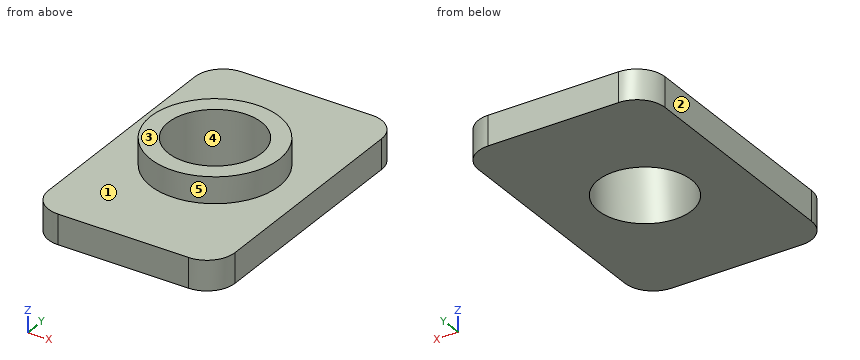
Autodesk Inventor part; units mm, degrees
ref_plane "YZ Plane" through (0, 0, 0) normal (1, 0, 0) x (0, 1, 0)
ref_plane "XZ Plane" through (0, 0, 0) normal (0, 1, 0) x (-1, 0, 0)
ref_plane "XY Plane" through (0, 0, 0) normal (0, 0, 1) x (1, 0, 0)
sketch "Sketch1" plane through (0, 0, 0) normal (0, 0, 1) x (1, 0, 0)
  line L0 (-5, 7.5) -> (5, 7.5)
  line L1 (5, 7.5) -> (5, -7.5)
  line L2 (5, -7.5) -> (-5, -7.5)
  line L3 (-5, -7.5) -> (-5, 7.5)
  line L4 (0, 7.5) -> (0, -7.5) construction
  line L5 (-5, 0) -> (5, 0) construction
  circle A0 centre (0, 0) radius 2.5
  dimension "d0" = 15
  dimension "d1" = 10
  dimension "d2" = 5
extrude "Extrusion1" add sketch "Sketch1" along normal blind 1.6
sketch "Sketch2" plane through (0, 0, 1.6) normal (0, 0, 1) x (1, 0, 0)
  circle A0 centre (0, 0) radius 2.5
  circle A1 centre (0, 0) radius 3.45
  dimension "d5" = 6.9
extrude "Extrusion2" add sketch "Sketch2" along normal blind 1.4
thread "Thread1"
fillet "Fillet1" radius 1.5 4 edges at (5, 7.5, 0.8) (-5, 7.5, 0.8) (-5, -7.5, 0.8) (5, -7.5, 0.8)
properties part number "t-nut"
Geometry check sheet. Reference: the model listing, model coordinates, mm. Face numbers are marked on the shaded views. A direction names the side the tool comes from. Coordinates: 2 decimals unless noted, no trailing zeros. Order: outer loops, then holes, each group sorted by start corner. A loop starts at its lowest first (then second) coordinate and runs counter-clockwise, first axis right, second up. Notation, with made-up numbers: M 65.25,60.5 L 72.25,60.5 A31 ccw 72.25,89.5 Z; hole C 45,63 d6. An arc over 180 degrees is marked long. Answer as a JSON object with one key per item and string values.
Q1. Tool access check on the marked faces 1 and 2. Record the directions out of +Z, -Z, +X, -X, +Y, -Y that give a thin tool (end or side, any length) a straight path to the whole face; none if there is none.
Results are:
{"face 1": "+Z", "face 2": "+Z, -Z, -X, +Y, -Y"}
Q2. Cross-section at C-C on z = 0.5. Record the cut outline in (x, y).
Results are:
{"outline": "M -5,-6 A1.5 ccw -3.5,-7.5 L 3.5,-7.5 A1.5 ccw 5,-6 L 5,6 A1.5 ccw 3.5,7.5 L -3.5,7.5 A1.5 ccw -5,6 Z; hole C 0,0 d5"}
Q3. Release check for a two-part mould opening along Y. For the marked faces 3, 4 and 5 record: released by +Y, released by -Y, zero draft, split by the parting line, or undercut.
Results are:
{"face 3": "zero draft", "face 4": "undercut", "face 5": "split by the parting line"}
Q4. Cross-section at D-D on y = -3. Record the cut outline in (x, z).
Results are:
{"outline": "M -5,0 L 5,0 L 5,1.6 L 1.7,1.6 L 1.7,3 L -1.7,3 L -1.7,1.6 L -5,1.6 Z"}
Q5. Scan lines: line 1 (Y direction, x = 0, z = 1.25); line 2 (Z direction, x = 0.5, y = -3.5); line 3 (Y direction, x = -2, z = 1.2). Record each from-to range of solid material in increasing order.
Results are:
{"line 1": "y = -7.5 to -2.5, 2.5 to 7.5", "line 2": "z = 0 to 1.6", "line 3": "y = -7.5 to -1.5, 1.5 to 7.5"}
Q6. Cross-section at A-A on y = 0. Record the cut outline in (x, z).
Results are:
{"outline": "M -5,0 L -2.5,0 L -2.5,3 L -3.45,3 L -3.45,1.6 L -5,1.6 Z; M 2.5,0 L 5,0 L 5,1.6 L 3.45,1.6 L 3.45,3 L 2.5,3 Z"}
Q7. Cross-section at B-B on x = 0. Record the cut outline in (y, z).
Results are:
{"outline": "M -7.5,0 L -2.5,0 L -2.5,3 L -3.45,3 L -3.45,1.6 L -7.5,1.6 Z; M 2.5,0 L 7.5,0 L 7.5,1.6 L 3.45,1.6 L 3.45,3 L 2.5,3 Z"}
